Part model, mm, in its own coordinate system. Face numbers are marked on the shaded views. A direction names the side the tool comes from. Round coordinates to 2 decimals unless told otherwise and drop trailing zeros. Order: outer loops, then holes, each group sorted by start corner. A loop starts at its lowest first (then second) coordinate and runs counter-clockwise, first axis right, second up. Notation, with made-up numbers: (-14, 85.25) - (-7, 85.25) arc R23 ccw to (-7, 121.25) - close; hole circle Ø10 at (0.25, -22). An arc over 180 degrees is marked (long way). Return JSON: item names as keys, results as strings. Group by question number.
Item 1: Drop flat-ended pins along their axis: pin 1 (8 mm diameter, centred on x = 23, z = 44, fed in from -Y); pin 2 (1.6 mm diameter, centred on x = 98.5, z = -10.5, fed in from -Y); pin 3 (8 mm diameter, centred on y = 27, z = -14, fed in from -X). Give the stop position or say it passes through.
Item 2: Saw through at B-B on x = 80. List the corners of the cut face in (y, z), and give its area (3 significant figures).
Item 3: Tool access for the marked faces 1 and 2: list every direction of +Z, -Z, +X, -X, +Y, -Y with a clear straight run to the whole face (end or side of a thin tool).
Item 4: Two-plate mould, pull along Z, no slides. Class the marked faces 3, 4, 5 and 6: released by +Z, released by -Z, zero draft, split by the parting line, or undercut.
Item 5: Saw through at A-A on z = 17. List the corners of the cut face in (x, y), and give its area (3 significant figures).
Item 6: Saw through at C-C on y = 37. State how many separate pieces and enclosed holes the cut face has, and give its area (3 significant figures).
Item 7: Probe probe 1 along X at (y, z) = (38.5, -44); probe 2 along X at (y, z) = (28, -31.5); probe 3 along Z at (x, y) = (-59, 17.5). List the from-to ranges inside material, lowest first.
Item 8: Saw through at D-D on z = 47.5. List the corners of the cut face in (x, y), and give its area (3 significant figures).
```python
from build123d import *

# Parameters (mm, degrees)
SKETCH_1_W           = 200
SKETCH_1_H           = 115
F_40MM_DEPTH         = 40
SHELL_3_T            = 1.5
SKETCH_2_W           = 165
SKETCH_2_H           = 100
CUT_EXTRUDE_7_DEPTH  = 1.5
SKETCH_3_W           = 16
SKETCH_3_H           = 10
CUT_EXTRUDE_8_DEPTH  = 1.5
SKETCH_4_W           = 23
SKETCH_4_H           = 12
CUT_EXTRUDE_9_DEPTH  = 1.5
EXTRUDE_1_DEPTH      = 13
EXTRUDE_2_DEPTH      = 2
FILLET_2_R           = 1
SKETCH_9_W           = 30
SKETCH_9_H           = 30
CUT_EXTRUDE_10_DEPTH = 10


with BuildPart() as part:
    # 草图1 → 凸台-拉伸40mm (new body)
    with BuildSketch(Plane(origin=(0, 0, 0), x_dir=(1, 0, 0), z_dir=(0, 1, 0))):
        Rectangle(SKETCH_1_W, SKETCH_1_H)
    extrude(amount=F_40MM_DEPTH)

    # 抽壳3
    shell_3_openings = [part.faces().sort_by_distance(p)[0] for p in [
        (0, 0, 0),
    ]]
    offset(amount=SHELL_3_T, openings=shell_3_openings, kind=Kind.INTERSECTION)

    # 草图2 → 切除-拉伸7 (cut)
    with BuildSketch(Plane(origin=(0, 40, 0), x_dir=(1, 0, 0), z_dir=(0, 1, 0))):
        Rectangle(SKETCH_2_W, SKETCH_2_H)
    extrude(amount=CUT_EXTRUDE_7_DEPTH, mode=Mode.SUBTRACT)

    # 草图3 → 切除-拉伸8 (cut)
    with BuildSketch(Plane(origin=(-100, 0, 0), x_dir=(0, 0, -1), z_dir=(1, 0, 0))):
        with Locations((12, 27.5)):
            Rectangle(SKETCH_3_W, SKETCH_3_H)
    extrude(amount=-CUT_EXTRUDE_8_DEPTH, mode=Mode.SUBTRACT)

    # 草图4 → 切除-拉伸9 (cut)
    with BuildSketch(Plane.ZY.offset(-100)):
        with Locations((0, 22.5)):
            Rectangle(SKETCH_4_W, SKETCH_4_H)
    extrude(amount=-CUT_EXTRUDE_9_DEPTH, mode=Mode.SUBTRACT)

    # 草图6 → 凸台-拉伸1 (add)
    with BuildSketch(Plane(origin=(0, 40, 0), x_dir=(-1, 0, 0), z_dir=(0, -1, 0))):
        Polygon((-95.25, 52.7), (-85.25, 52.7), (-85.25, 54.2), (-96.75, 54.2), (-96.75, 42.7), (-95.25, 42.7), align=None)
        Polygon((-96.75, -42.7), (-95.25, -42.7), (-95.25, -52.7), (-85.25, -52.7), (-85.25, -54.2), (-96.75, -54.2), align=None)
        Polygon((85.25, -52.7), (85.25, -54.2), (96.75, -54.2), (96.75, -42.7), (95.25, -42.7), (95.25, -52.7), align=None)
        Polygon((85.25, 52.7), (85.25, 54.2), (96.75, 54.2), (96.75, 42.7), (95.25, 42.7), (95.25, 52.7), align=None)
    extrude(amount=EXTRUDE_1_DEPTH)

    # 草图7 → 凸台-拉伸2 (add)
    with BuildSketch(Plane.ZY.offset(-100)):
        Polygon((-7.5, 28.5), (-7.5, 30), (-13, 30), (-13, 24.5), (-11.5, 24.5), (-11.5, 28.5), align=None)
        Polygon((7.5, 28.5), (7.5, 30), (13, 30), (13, 24.5), (11.5, 24.5), (11.5, 28.5), align=None)
        Polygon((7.5, 16.5), (7.5, 15), (13, 15), (13, 20.5), (11.5, 20.5), (11.5, 16.5), align=None)
        Polygon((-13, 20.5), (-11.5, 20.5), (-11.5, 16.5), (-7.5, 16.5), (-7.5, 15), (-13, 15), align=None)
    extrude(amount=EXTRUDE_2_DEPTH)

    # 圆角2
    fillet_2_edges = [part.edges().sort_by_distance(p)[0] for p in [
        (101.5, 41.5, 0),
        (0, 41.5, -59),
        (100, 20, 57.5),
        (-101.5, 41.5, 0),
        (-101.5, 20.75, -59),
        (101.5, 20.75, -59),
        (-101.5, 20.75, 59),
        (0, 41.5, 59),
    ]]
    fillet(fillet_2_edges, radius=FILLET_2_R)

    # 草图9 → 切除-拉伸10 (cut)
    with BuildSketch(Plane(origin=(0, 0, 57.5), x_dir=(-1, 0, 0), z_dir=(0, 0, -1))):
        Rectangle(SKETCH_9_W, SKETCH_9_H)
    extrude(amount=-CUT_EXTRUDE_10_DEPTH, mode=Mode.SUBTRACT)


solid = part.part
```
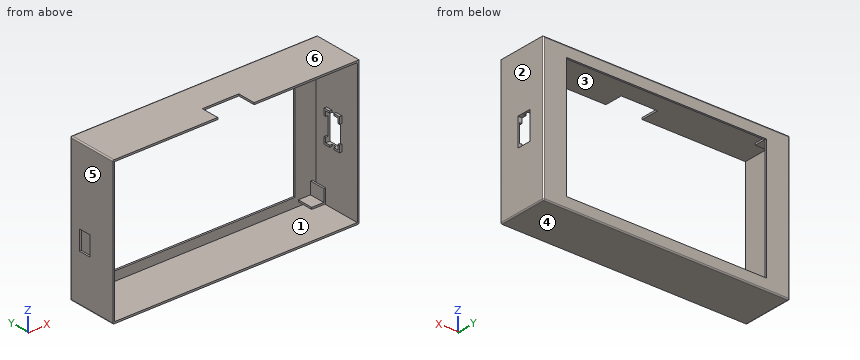
Filled in:
{
 "1": {"pin 1": "passes through", "pin 2": "stops at y = 15", "pin 3": "stops at x = 98"},
 "2": {"outline": "(0, -59) - (40.5, -59) arc R1 ccw to (41.5, -58) - (41.5, -50) - (40, -50) - (40, -57.5) - (0, -57.5) - close; (0, 57.5) - (40, 57.5) - (40, 50) - (41.5, 50) - (41.5, 58) arc R1 ccw to (40.5, 59) - (0, 59) - close", "area": "147 mm^2"},
 "3": {"face 1": "-Y", "face 2": "+Z, -Z, +X, +Y, -Y"},
 "4": {"face 3": "undercut", "face 4": "released by -Z", "face 5": "zero draft", "face 6": "released by +Z"},
 "5": {"outline": "(-101.5, 0) - (-100, 0) - (-100, 40) - (-82.5, 40) - (-82.5, 41.5) - (-100.5, 41.5) arc R1 ccw to (-101.5, 40.5) - close; (82.5, 40) - (100, 40) - (100, 0) - (101.5, 0) - (101.5, 40.5) arc R1 ccw to (100.5, 41.5) - (82.5, 41.5) - close", "area": "177 mm^2"},
 "6": {"separate pieces": "5", "enclosed holes": "1", "area": "1,080 mm^2"},
 "7": {"probe 1": "x = -101.5 to -100, -96.75 to -95.25, 95.25 to 96.75, 100 to 101.5", "probe 2": "x = -101.5 to -100, 100 to 101.5", "probe 3": "z = -59 to -57.5, 57.5 to 59"},
 "8": {"outline": "(-101.5, 0) - (-100, 0) - (-100, 40) - (-96.75, 40) - (-96.75, 27) - (-95.25, 27) - (-95.25, 40) - (-82.5, 40) - (-82.5, 41.5) - (-100.5, 41.5) arc R1 ccw to (-101.5, 40.5) - close; (82.5, 40) - (95.25, 40) - (95.25, 27) - (96.75, 27) - (96.75, 40) - (100, 40) - (100, 0) - (101.5, 0) - (101.5, 40.5) arc R1 ccw to (100.5, 41.5) - (82.5, 41.5) - close", "area": "216 mm^2"}
}
